Input: dimensioned drawing with shaded views. Units: mm. Origin: part minimum x, y, z. A direction names the side the tool comes from. Give positions to 0.01 mm unless a question says otherwise; leave off trailing zeros. Write each loop counter-clockwise with the first axis right and the second up, starting at its lowest first coordinate (ties: lowest second). Pieces come first, ordered by that corner, then holes.
Q1. Pin query (flat end, axial travel): pin 1 Ø11.5 at (x, z) = (20, 10) entering from +Y; pin 2 Ø9 at (y, z) = (25.5, 37.5) entering from -X; pin 3 Ø1.5 at (y, z) = (16, 27) entering from +X; pin 4 Ø9 at (y, z) = (30, 30) entering from -X. Return the tip coordinate at first contact, or that it passes through.
Q2. Reachability of the marked faces 1, 2 and 3 from +Z, -Z, +X, -X, +Y, -Y: full face, straight path, thin tool, end or side. Return the list, or none.
Q3. Section C-C (z = 53). Return the cut outline in (x, y), plus the area to 3 significant figures.
Q4. Section D-D (z = 41.5). Return the cut outline in (x, y), plus the area to 3 significant figures.
Q5. Line query: line 1 (Z direction, x = 20, y = 3.1); line 2 (X direction, y = 46, z = 30); line 3 (X direction, y = 19.5, z = 45.5). Output: solid intervals per line, ascending.
Q6. Section A-A (x = 95). Return the cut outline in (y, z), plus the area to 3 significant figures.
Q7. Section B-B (y = 30). Return the cut outline in (x, z).
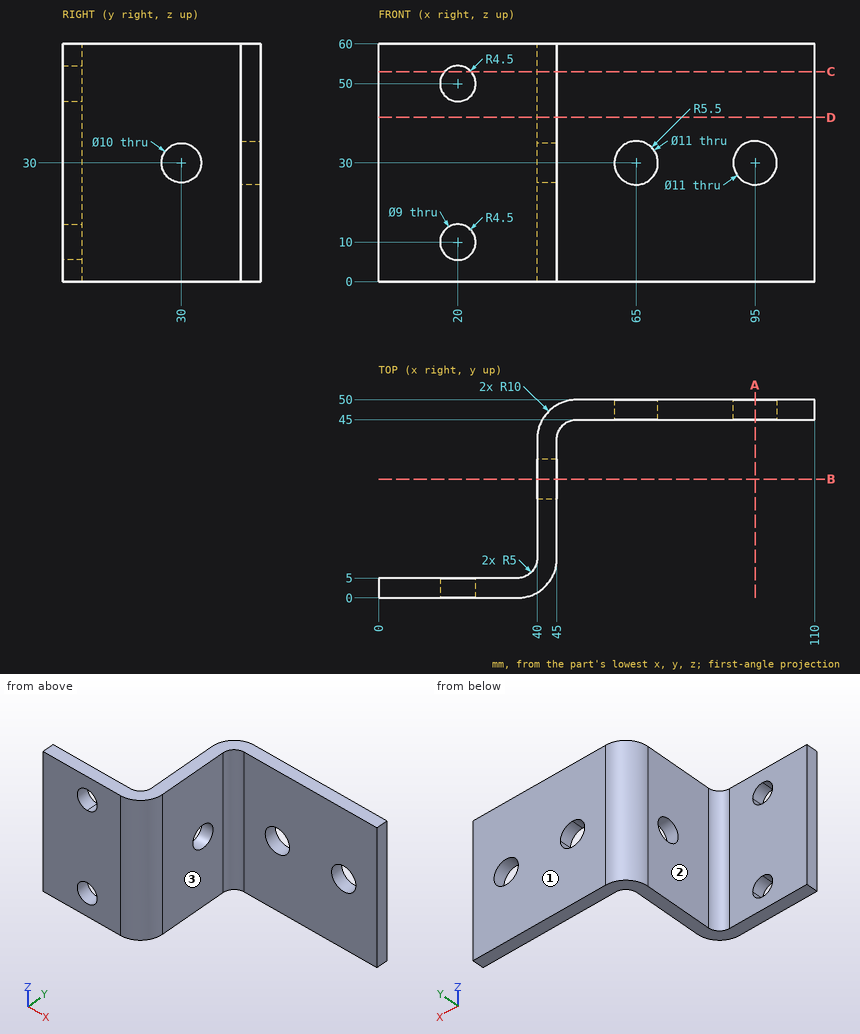
Computed:
1. pin 1: stops at y = 5
1. pin 2: stops at x = 40
1. pin 3: stops at x = 45
1. pin 4: passes through
2. face 1: +Z, -Z, +X, -X, +Y
2. face 2: +Z, -Z, -X, +Y
2. face 3: +Z, -Z, +X, -Y
3. outline: (0, 0) - (16.65, 0) - (16.65, 5) - (0, 5) - close; (23.35, 0) - (35, 0) arc R10 ccw to (45, 10) - (45, 40) arc R5 cw to (50, 45) - (110, 45) - (110, 50) - (50, 50) arc R10 ccw to (40, 40) - (40, 10) arc R5 cw to (35, 5) - (23.35, 5) - close
3. area: 709 mm2
4. outline: (0, 0) - (35, 0) arc R10 ccw to (45, 10) - (45, 40) arc R5 cw to (50, 45) - (110, 45) - (110, 50) - (50, 50) arc R10 ccw to (40, 40) - (40, 10) arc R5 cw to (35, 5) - (0, 5) - close
4. area: 743 mm2
5. line 1: z = 0 to 5.5, 14.5 to 45.5, 54.5 to 60
5. line 2: x = 42 to 59.5, 70.5 to 89.5, 100.5 to 110
5. line 3: x = 40 to 45
6. outline: (45, 0) - (50, 0) - (50, 24.5) - (45, 24.5) - close; (45, 35.5) - (50, 35.5) - (50, 60) - (45, 60) - close
6. area: 245 mm2
7. outline: (40, 0) - (45, 0) - (45, 25) - (40, 25) - close; (40, 35) - (45, 35) - (45, 60) - (40, 60) - close
